```python
from build123d import *

# Parameters (mm, degrees)
PAD006_DEPTH        = 16
FILLET005_R         = 2.5
HOLE006_D           = 4.5
HOLE006_CBORE_D     = 5.6
HOLE006_CBORE_DEPTH = 4.4
PAD009_DEPTH        = 4
SKETCH027_R         = 16.8
PAD010_DEPTH        = 8


with BuildPart() as part:
    # Sketch023 → Pad006 (new body)
    with BuildSketch(Plane.XY):
        with BuildLine():
            Line((-4.795832, 11), (-21, 11))
            Line((-21, 11), (-21, 8))
            Line((-21, 8), (-4.123106, 8))
            ThreePointArc((-4.123106, -8), (9, 0), (-4.123106, 8))
            Line((-21, -8), (-4.123106, -8))
            Line((-21, -12), (-21, -8))
            Line((0, -12), (-21, -12))
            ThreePointArc((0, -12), (11.74734, 2.44949), (-4.795832, 11))
        make_face()
    extrude(amount=PAD006_DEPTH)

    # Fillet005
    fillet005_edges = [part.edges().sort_by_distance(p)[0] for p in [
        (-21, 9.5, 0),
        (-21, 9.5, 16),
        (-21, -10, 16),
        (-21, -10, 0),
    ]]
    fillet(fillet005_edges, radius=FILLET005_R)

    # Hole006 (through all)
    with Locations(Plane.XZ.offset(12)):
        with Locations((-13, 8)):
            CounterBoreHole(HOLE006_D / 2, HOLE006_CBORE_D / 2, HOLE006_CBORE_DEPTH)

    # Sketch028 → Pad009 (join)
    with BuildSketch(Plane.XY):
        with BuildLine():
            Line((14.620192, 2.5), (34.237617, 2.5))
            ThreePointArc((34.237617, 2.5), (35.379237, 1.134862), (37, 0.4))
            Line((37, 0.4), (37, -0.4))
            ThreePointArc((37, -0.4), (35.379237, -1.134862), (34.237617, -2.5))
            Line((14.620192, -2.5), (34.237617, -2.5))
            ThreePointArc((14.620192, -2.5), (12.440742, -3.145898), (10.965144, -4.875))
            Line((10.965144, 4.875), (10.965144, -4.875))
            ThreePointArc((10.965144, 4.875), (12.440742, 3.145898), (14.620192, 2.5))
        make_face()
    extrude(amount=PAD009_DEPTH)

    # Sketch027 → Pad010 (join)
    with BuildSketch(Plane.XY):
        with BuildLine():
            ThreePointArc((19.174457, -2.5), (55, 0), (19.174457, 2.5))
            Line((19.174457, 2.5), (14.620192, 2.5))
            ThreePointArc((10.965144, 4.875), (12.440742, 3.145898), (14.620192, 2.5))
            Line((10.965144, 4.875), (10.965144, -4.875))
            ThreePointArc((14.620192, -2.5), (12.440742, -3.145898), (10.965144, -4.875))
            Line((19.174457, -2.5), (14.620192, -2.5))
        make_face()
        with Locations((37, 0)):
            Circle(SKETCH027_R, mode=Mode.SUBTRACT)
    extrude(amount=PAD010_DEPTH)


solid = part.part
```
Geometry check sheet. Reference: the model listing, model coordinates, mm. A direction names the side the tool comes from. Give positions to 0.01 mm unless a question says otherwise; leave off trailing zeros. Write each loop counter-clockwise with the first axis right and the second up, starting at its lowest first coordinate (ties: lowest second). Pieces come first, ordered by that corner, then holes. Notation, with made-up numbers: (7, 47) -> (36, 47) arc R15 cw to (36, 57) -> close; hole circle Ø10 at (-23.5, 9.25). An arc over 180 degrees is marked (long way). One line per question, with ' | ' between items.
Item 1: Scan lines: line 1 along X through (y, z) = (0, 6.5); line 2 along X through (y, z) = (-4.5, 6.5); line 3 along Y through (x, z) = (37, 6.25). Record each from-to range of solid material in increasing order.
Determined:
line 1: 9 to 20.2, 53.8 to 55 | line 2: 7.79 to 11.16, 19.57 to 20.81, 53.19 to 54.43 | line 3: -18 to -16.8, 16.8 to 18
Item 2: Depth check by flat-ended pin: pin 1 (6 mm diameter, centred on y = 4.5, z = 6.5, fed in from +X); pin 2 (0.9 mm diameter, centred on y = 0, z = 3, fed in from +X); pin 3 (1 mm diameter, centred on x = 45, z = 7, fed in from -Y); pin 4 (4 mm diameter, centred on x = -4, y = 5.5, fed in from -Z). Enter the tip coordinate at first touch or a pass-through.
Determined:
pin 1: x = 54.94 | pin 2: x = 55 | pin 3: y = -16.36 | pin 4: through
Item 3: Sectioned sample at B-B, the plane y = 10. Record the boundary of the cut face in (x, z), plus the area to 3 significant figures.
Determined:
outline: (-21, 2.5) arc R2.5 ccw to (-18.5, 0) -> (6.63, 0) -> (6.63, 16) -> (-18.5, 16) arc R2.5 ccw to (-21, 13.5) -> close; (22.03, 0) -> (23.5, 0) -> (23.5, 8) -> (22.03, 8) -> close; (50.5, 0) -> (51.97, 0) -> (51.97, 8) -> (50.5, 8) -> close; hole circle Ø4.5 at (-13, 8) | area: 447 mm^2
Item 4: Sectioned sample at A-A, the plane x = -13. Record the boundary of the cut face in (y, z), plus the area to 3 significant figures.
Determined:
outline: (-12, 0) -> (-8, 0) -> (-8, 5.2) -> (-12, 5.2) -> close; (-12, 10.8) -> (-8, 10.8) -> (-8, 16) -> (-12, 16) -> close; (8, 0) -> (11, 0) -> (11, 5.75) -> (8, 5.75) -> close; (8, 10.25) -> (11, 10.25) -> (11, 16) -> (8, 16) -> close | area: 76.1 mm^2
Item 5: Sectioned sample at C-C, the plane x = 41.5. Record the boundary of the cut face in (y, z), plus the area to 3 significant figures.
Determined:
outline: (-17.43, 0) -> (-16.19, 0) -> (-16.19, 8) -> (-17.43, 8) -> close; (16.19, 0) -> (17.43, 0) -> (17.43, 8) -> (16.19, 8) -> close | area: 19.9 mm^2
Item 6: Access from +Z, -Z, +X, -X, +Y, -Y to the whole of each face (thin tool, end or side, straight path). Record for faces 1 (the flat face through (-13, -8, 4)), 2 (the cylindrical face through (-13.607, -10.028, 5.267)), 3 (the cylindrical face through (12.468, -3.128, 3.944)), 4 (the cylindrical face through (35.36, 1.15, 1.97)).
Determined:
face 1: +Z, -Z, -X | face 2: -Y | face 3: +Z, -Z, -Y | face 4: +Z, -Z
Item 7: Sectioned sample at D-D, the plane z = 12.25. Record the boundary of the cut face in (x, y), plus the area to 3 significant figures.
Determined:
outline: (-21, -12) -> (0, -12) arc R12 ccw (long way) to (-4.8, 11) -> (-21, 11) -> (-21, 8) -> (-4.12, 8) arc R9 cw (long way) to (-4.12, -8) -> (-21, -8) -> close | area: 244 mm^2
Item 8: Draft check along Y on faces 5 (the flat face through (17, 2.5, 4)), 6 (the flat face through (-15, 8, 10)), 7 (the flat face through (-10, -12, 6)). Enter one of: released by +Y, released by -Y, zero draft, split by the parting line, or undercut.
Determined:
face 5: released by +Y | face 6: undercut | face 7: released by -Y
